Can you work these out from the model? Positions are in its coordinate system, mm. Coordinates: 2 decimals unless noted, no trailing zeros. Loops run counter-clockwise (first coordinate to the right, second up) from the corner with the lowest first, then second, coordinate; pieces in that order, holes last.
```python
from build123d import *

# Parameters (mm, degrees)
SKETCH2_R           = 3.175
BOSS_EXTRUDE1_DEPTH = 1.905


with BuildPart() as part:
    # Sketch2 → Boss-Extrude1 (new body)
    with BuildSketch(Plane(origin=(0, 0, 0), x_dir=(1, 0, 0), z_dir=(0, 1, 0))):
        with BuildLine():
            Line((-24.183512242, 17.960512242), (-24.183512242, 3.75))
            Line((-24.183512242, 3.75), (-10, 3.75))
            Line((-10, 3.75), (-10, 10))
            Line((-10, 10), (30, 10))
            Line((30, 10), (30, -10))
            Line((30, -10), (11.737512242, -10))
            Line((11.737512242, -10), (10, -10))
            Line((10, -10), (0, -10))
            Line((0, -10), (-10, -10))
            Line((-10, -10), (-10, -3.75))
            Line((-10, -3.75), (-24.183512242, -3.75))
            Line((-24.183512242, -3.75), (-36.000215624, -3.75))
            ThreePointArc((-36.000215624, -3.75), (8.539491503, -35.173215802), (33.7119771, 13.175))
            Line((33.7119771, 13.175), (-13.982497463, 13.175))
            ThreePointArc((-13.982497463, 13.175), (-12.326645232, 15.317545819), (-11.737512242, 17.960512242))
            ThreePointArc((-11.737512242, 17.960512242), (-13.560186743, 22.360837741), (-17.960512242, 24.183512242))
            ThreePointArc((-17.960512242, 24.183512242), (-22.360837741, 22.360837741), (-24.183512242, 17.960512242))
        make_face()
        with Locations((-17.960512242, 17.960512242)):
            Circle(SKETCH2_R, mode=Mode.SUBTRACT)
        with Locations((17.960512242, -17.960512242)):
            Circle(SKETCH2_R, mode=Mode.SUBTRACT)
    extrude(amount=BOSS_EXTRUDE1_DEPTH)


solid = part.part
```
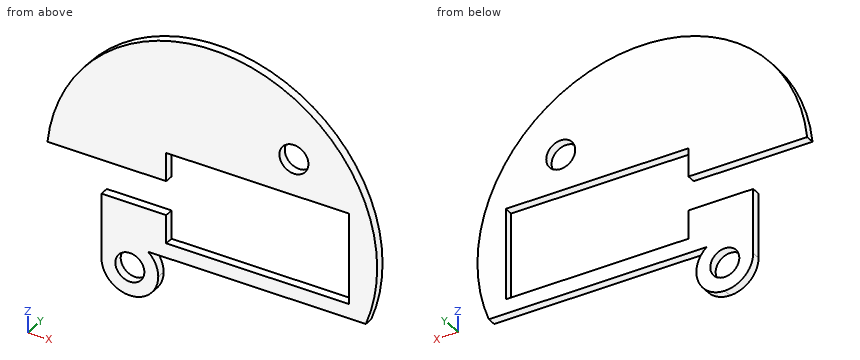
(1) I'm going to push flat-ended pins straight in: pin 1 (2 mm diameter, centred on x = 13.5, z = -8, fed in from -Y); pin 2 (10 mm diameter, centred on x = 17.96, z = 17.96, fed in from -Y); pin 3 (0.6 mm diameter, centred on x = 0, y = 1.5, fed in from -Z) (3 decimals). Where does each tip first touch, or does it pass through?
Check values:
pin 1: passes through
pin 2: stops at y = 0
pin 3: stops at z = -13.175
(2) I want a section at C-C on y = 0.7. State how many separate pieces and enclosed holes the cut face has, then the cut area to 3 significant figures.
Check values:
separate pieces: 1
enclosed holes: 2
area: 1,950 mm2
(3) I want a section at A-A on z = 8. Write out the boundary of the cut face in (x, y) (3 decimals).
Check values:
outline: (-35.3, 0) - (-10, 0) - (-10, 1.905) - (-35.3, 1.905) - close; (30, 0) - (35.3, 0) - (35.3, 1.905) - (30, 1.905) - close
(4) I want a section at D-D on z = 0. Write out the boundary of the cut face in (x, y) (3 decimals), then the cut area to 3 significant figures.
Check values:
outline: (30, 0) - (36.195, 0) - (36.195, 1.905) - (30, 1.905) - close
area: 11.8 mm2
(5) I want a section at B-B on x = 0. Write out the boundary of the cut face in (y, z) (3 decimals), then the cut area to 4 significant figures.
Check values:
outline: (0, -13.175) - (1.905, -13.175) - (1.905, -10) - (0, -10) - close; (0, 10) - (1.905, 10) - (1.905, 36.195) - (0, 36.195) - close
area: 55.95 mm2
(6) If I drill on probe 1 along Z at (x, y) = (-19, 1.55); probe 2 along Z at (x, y) = (18, 1) (3 decimals); probe 3 along Z at (x, y) = (-4, 1.25) (3 decimals), over which ranges is the centre line in solid material (lowest first)?
Check values:
probe 1: z = -24.1 to -20.96, -14.96 to -3.75, 3.75 to 30.81
probe 2: z = -13.175 to -10, 10 to 14.786, 21.135 to 31.402
probe 3: z = -13.175 to -10, 10 to 35.973
